```python
from build123d import *

# Parameters (mm, degrees)
F0_W     = 1
F0_H     = 1
F1_DEPTH = 12
F2_R     = 0.4
F3_DEPTH = 2.15
F4_SIZE  = 0.25


with BuildPart() as f1:
    # F0 (on Top) → F1 (new body)
    with BuildSketch(Plane.XY):
        with Locations((0.5, 0.5)):
            Rectangle(F0_W, F0_H)
    extrude(amount=F1_DEPTH)

    # F2 (on face) → F3 (join)
    with BuildSketch(Plane.XY.offset(12)):
        with Locations((0.5, 0.5)):
            Circle(F2_R)
    extrude(amount=F3_DEPTH)

    # F4
    f4_edges = [f1.edges().sort_by_distance(p)[0] for p in [
        (0.5, 0, 0),
        (0, 0.5, 0),
        (1, 0.5, 0),
        (0.5, 1, 0),
    ]]
    chamfer(f4_edges, length=F4_SIZE)


solid = f1.part
```
Can you work these out from the model? Positions are in its coordinate system, mm. Coordinates: 2 decimals unless noted, no trailing zeros. Loops run counter-clockwise (first coordinate to the right, second up) from the corner with the lowest first, then second, coordinate; pieces in that order, holes last.
Item 1: Please list where these lines run through material, in increasing order: L1, parallel to Z at x = 0.85, y = 0.2; L2, parallel to X at y = 0.6, z = 13; L3, parallel to Z at x = 0.2, y = 0.65.
Answers below:
L1: z = 0.1 to 12
L2: x = 0.11 to 0.89
L3: z = 0.05 to 14.15
Item 2: Suppose I cut it at A-A (x = 0.5). Please give me the cut outline in (y, z).
Answers below:
outline: (0, 0.25) - (0.25, 0) - (0.75, 0) - (1, 0.25) - (1, 12) - (0.9, 12) - (0.9, 14.15) - (0.1, 14.15) - (0.1, 12) - (0, 12) - close
